Can you work these out from the model? Positions are in its coordinate system, mm. A direction names the side the tool comes from. Round coordinates to 2 decimals unless told otherwise and drop trailing zeros. Loops run counter-clockwise (first coordinate to the right, second up) from the corner with the lowest first, then second, coordinate; pieces in that order, holes last. Notation, with made-up numbers: (-7, -5) - (41, -5) arc R22 cw to (41, 23) - close; hole circle Ø11 at (48, 74.5). An arc over 180 degrees is marked (long way). Answer as CSV lines item,"result".
```python
from build123d import *

# Parameters (mm, degrees)
F1_DEPTH = 480
F3_DEPTH = 50
F5_DEPTH = 25
F7_DEPTH = 25


with BuildPart() as f1:
    # F0 (on Front) → F1 (new body)
    with BuildSketch(Plane.XZ):
        Polygon((-161, 0), (0, 0), (161, 0), (302.421356, 141.421356), (299.592929, 144.249783), (159.343146, 4), (0, 4), (-159.343146, 4), (-299.592929, 144.249783), (-302.421356, 141.421356), align=None)
    extrude(amount=F1_DEPTH)

    # F2 (on face) → F3 (join)
    with BuildSketch(Plane.XZ.offset(480)):
        Polygon((-299.592929, 144.249783), (-302.421356, 141.421356), (-161, 0), (161, 0), (302.421356, 141.421356), (299.592929, 144.249783), (159.343146, 4), (-159.343146, 4), align=None)
    extrude(amount=F3_DEPTH)

    # F4 (on face) → F5 (cut)
    with BuildSketch(Plane(origin=(-77.671573, 0, -77.671573), x_dir=(0, 1, 0), z_dir=(0.707107, 0, 0.707107))):
        with BuildLine():
            Line((-754.76669, 313.844192), (-530, 115.501046))
            ThreePointArc((-530, 115.501046), (-474.376217, 207.819426), (-455, 313.844192))
            Line((-455, 313.844192), (-754.76669, 313.844192))
        make_face()
    extrude(amount=-F5_DEPTH, mode=Mode.SUBTRACT)

    # F6 (on face) → F7 (cut)
    with BuildSketch(Plane(origin=(77.671573, 0, -77.671573), x_dir=(0, -1, 0), z_dir=(-0.707107, 0, 0.707107))):
        with BuildLine():
            Line((754.76669, 313.844192), (455, 313.844192))
            ThreePointArc((455, 313.844192), (474.376217, 207.819426), (530, 115.501046))
            Line((530, 115.501046), (754.76669, 313.844192))
        make_face()
    extrude(amount=-F7_DEPTH, mode=Mode.SUBTRACT)


solid = f1.part
```
Q1. Imagine slicing it at A-A (y = -161.5). Write out the boundary of the cut face in (x, z).
Checks:
outline,"(-302.42, 141.42) - (-161, 0) - (161, 0) - (302.42, 141.42) - (299.59, 144.25) - (159.34, 4) - (-159.34, 4) - (-299.59, 144.25) - close"
Q2. On a 3-axis mill with a long thin cutter (end or side, diameter ignored), from which of +Z, -Z, +X, -X, +Y, -Y can I reach the whole of each face in a straight line? I mean faces 1 (the flat face through (-228.486, -261.29, 73.143)), 2 (the cylindrical face through (-225.01, -474.92, 66.88)). Say none if no direction works.
Checks:
face 1,"+Z, +Y, -Y"
face 2,"+Z, -X, -Y"
Q3. I'm going to push flat-ended pins straight in: pin 1 Ø1 at (y, z) = (-315.5, 42.5) entering from -X; pin 2 Ø8 at (x, y) = (-96, -470) entering from +Z; pin 3 Ø12 at (y, z) = (-455, 59) entering from +X. Where does each tip first touch, or does it pass through?
Checks:
pin 1,"x = -204"
pin 2,"z = 4"
pin 3,"x = 226"
Q4. Imagine slicing it at B-B (x = -23). Write out the boundary of the cut face in (y, z), then the cut area to 3 significant figures.
Checks:
outline,"(-530, 0) - (0, 0) - (0, 4) - (-530, 4) - close"
area,"2,120 mm²"
Q5. We'd pull the mould along X, two halves only. Please class faces 3 (the cylindrical face through (227.021, -473.843, 68.889)), 4 (the flat face through (-1, 0, 3)), 5 (the flat face through (2, -261, 4)), 6 (the flat face through (230.45, -261.29, 75.107)): pulls with the +X half, pulls with the -X half, needs draft (parallel to the pull), parting line crosses it, or undercut.
Checks:
face 3,"pulls with the +X half"
face 4,"needs draft"
face 5,"undercut"
face 6,"undercut"
Q6. If I drill on line 1 along Z through (x, y) = (18, -293.5); line 2 along X through (y, z) = (-269, 72); line 3 along X through (y, z) = (-49, 62.5), over which ranges is the centre line in solid material (lowest first)? Write a range as [from, to].
Checks:
line 1,"[0, 4]"
line 2,"[-233, -227.34], [227.34, 233]"
line 3,"[-223.5, -217.84], [217.84, 223.5]"
